Can you work these out from the model? Positions are in its coordinate system, mm. A direction names the side the tool comes from. Give positions to 0.01 mm unless a question says otherwise; leave off trailing zeros. Write each loop counter-clockwise with the first axis right and the second up, starting at its lowest first coordinate (ties: lowest second). Pieces come first, ordered by that corner, then holes. Notation, with made-up numbers: (66, 1.5) -> (97, 1.5) arc R29 cw to (97, 40.5) -> close; hole circle Ø2 at (88.5, 69). An arc over 180 degrees is marked (long way). One line per item, written item: value.
from build123d import *

# Parameters (mm, degrees)
SKETCH_W        = 77.5
SKETCH_H        = 50
PAD_DEPTH       = 5
SKETCH001_W     = 5
SKETCH001_H     = 50
PAD001_DEPTH    = 33
SKETCH002_W     = 50
SKETCH002_H     = 5
PAD002_DEPTH    = 6
SKETCH003_W     = 50
SKETCH003_H     = 5
PAD003_DEPTH    = 6
SKETCH004_R     = 2.5
POCKET_DEPTH    = 5.001
SKETCH005_R     = 5
POCKET001_DEPTH = 33
CHAMFER_SIZE    = 1
CHAMFER001_SIZE = 1
CHAMFER002_SIZE = 1


with BuildPart() as part:
    # Sketch → Pad (new body)
    with BuildSketch(Plane.XY):
        Rectangle(SKETCH_W, SKETCH_H)
    extrude(amount=PAD_DEPTH)

    # Sketch001 (on Face6 of Pad) → Pad001 (join)
    with BuildSketch(Plane.XY.offset(5)):
        with Locations((-36.25, 0)):
            Rectangle(SKETCH001_W, SKETCH001_H)
        with Locations((36.25, 0)):
            Rectangle(SKETCH001_W, SKETCH001_H)
    extrude(amount=PAD001_DEPTH)

    # Sketch002 (on Face10 of Pad001) → Pad002 (join)
    with BuildSketch(Plane.YZ.offset(38.75)):
        with Locations((0, 35.5)):
            Rectangle(SKETCH002_W, SKETCH002_H)
    extrude(amount=PAD002_DEPTH)

    # Sketch003 (on Face9 of Pad002) → Pad003 (join)
    with BuildSketch(Plane(origin=(-38.75, 0, 0), x_dir=(0, -1, 0), z_dir=(-1, 0, 0))):
        with Locations((0, 35.5)):
            Rectangle(SKETCH003_W, SKETCH003_H)
    extrude(amount=PAD003_DEPTH)

    # Sketch004 (on Face19 of Pad003) → Pocket (cut, through all)
    with BuildSketch(Plane(origin=(0, 0, 33), x_dir=(1, 0, 0), z_dir=(0, 0, -1))):
        with Locations((40.036056, -0.059049)):
            Circle(SKETCH004_R)
        with Locations((-40.036056, 0.059049)):
            Circle(SKETCH004_R)
    extrude(amount=-POCKET_DEPTH, mode=Mode.SUBTRACT)

    # Sketch005 (on Face4 of Pocket) → Pocket001 (cut)
    with BuildSketch(Plane(origin=(0, 0, 0), x_dir=(1, 0, 0), z_dir=(0, 0, -1))):
        with Locations((39.75, 0)):
            Circle(SKETCH005_R)
        with Locations((-39.75, 0)):
            Circle(SKETCH005_R)
    extrude(amount=-POCKET001_DEPTH, mode=Mode.SUBTRACT)

    # Chamfer
    chamfer_edges = [part.edges().sort_by_distance(p)[0] for p in [
        (0, 25, 0),
        (0, -25, 0),
        (-38.75, 14.94949, 0),
        (-38.75, -14.94949, 0),
        (38.75, -14.94949, 0),
        (38.75, 14.94949, 0),
    ]]
    chamfer(chamfer_edges, length=CHAMFER_SIZE)

    # Chamfer001
    chamfer001_edges = [part.edges().sort_by_distance(p)[0] for p in [
        (-44.75, 12.5, 33),
        (-44.75, -12.5, 33),
        (44.75, -12.5, 33),
        (44.75, 12.5, 33),
        (-41.75, -25, 33),
        (-41.75, 25, 33),
        (41.75, 25, 33),
        (41.75, -25, 33),
    ]]
    chamfer(chamfer001_edges, length=CHAMFER001_SIZE)

    # Chamfer002
    chamfer002_edges = [part.edges().sort_by_distance(p)[0] for p in [
        (-38.75, 25, 19),
        (-38.75, -25, 19),
        (38.75, 25, 19),
        (38.75, -25, 19),
    ]]
    chamfer(chamfer002_edges, length=CHAMFER002_SIZE)


solid = part.part
1) If we section it at B-B (x = -8): Write out the boundary of the cut face in (y, z).
Answer list:
outline: (-25, 1) -> (-24, 0) -> (24, 0) -> (25, 1) -> (25, 5) -> (-25, 5) -> close
2) I need wall thicknesses on L1, parallel to X at y = -21.5, z = 31; L2, parallel to Z at x = 18, y = -13. Which ranges of each line are inside material? Lowest first, please.
Answer list:
L1: x = -38.75 to -33.75, 33.75 to 38.75
L2: z = 0 to 5
3) For faces 4 (the face through (0, 0, 5)), 5 (the face through (38.75, 14, 17)), 6 (the face through (0, -25, 4)), 7 (the face through (-38.75, 14, 17)), 8 (the face through (34.75, -0.1, 16.27)), which set-ups out of +Z, -Z, +X, -X, +Y, -Y let a thin tool reach every point of the face, with its end or its side?
Answer list:
face 4: +Z, +Y, -Y
face 5: -Z, +X, +Y, -Y
face 6: +Z, -Z, +X, -X, -Y
face 7: -Z, -X, +Y, -Y
face 8: -Z, +X
4) If we section it at C-C (y = 15): Write out the boundary of the cut face in (x, z), and give its area (4 significant figures).
Answer list:
outline: (-44.75, 34) -> (-43.75, 33) -> (-38.75, 33) -> (-38.75, 1) -> (-37.75, 0) -> (37.75, 0) -> (38.75, 1) -> (38.75, 33) -> (43.75, 33) -> (44.75, 34) -> (44.75, 38) -> (33.75, 38) -> (33.75, 5) -> (-33.75, 5) -> (-33.75, 38) -> (-44.75, 38) -> close
area: 775.5 mm^2
5) We'd pull the mould along Y, two halves only. Please class faces 1 (the face through (-34.75, 0.1, 16.27)), 2 (the face through (38.75, -15, 17)), 3 (the face through (0, 25, 4)): released by +Y, released by -Y, zero draft, split by the parting line, or undercut.
Answer list:
face 1: undercut
face 2: zero draft
face 3: released by +Y
6) If we section it at A-A (z = 29.5): Write out the boundary of the cut face in (x, y).
Answer list:
outline: (-38.75, -24) -> (-37.75, -25) -> (-33.75, -25) -> (-33.75, 25) -> (-37.75, 25) -> (-38.75, 24) -> (-38.75, 4.9) arc R5 cw to (-38.75, -4.9) -> close; (33.75, -25) -> (37.75, -25) -> (38.75, -24) -> (38.75, -4.9) arc R5 cw to (38.75, 4.9) -> (38.75, 24) -> (37.75, 25) -> (33.75, 25) -> close
7) Will these pins go through, and if not, where does the flat tip stop? pin 1 (9.5 mm diameter, centred on y = 11, z = 15.5, fed in from -X); pin 2 (6.5 mm diameter, centred on x = -40.04, y = -0.06, fed in from -Z); pin 3 (10 mm diameter, centred on y = -12.5, z = 23, fed in from +X).
Answer list:
pin 1: stops at x = -38.75
pin 2: stops at z = 33
pin 3: stops at x = 38.75
